from build123d import *

# Parameters (mm, degrees)
CUT_EXTRUDE_START   = -25
CUT_EXTRUDE_1_DEPTH = 25
SKETCH_3_W          = 3.2
SKETCH_3_H          = 16
CUT_EXTRUDE_2_DEPTH = 4
SKETCH_4_R          = 1.6
CUT_EXTRUDE_3_DEPTH = 10


with BuildPart() as part:
    # 草图1 → 旋转1 (revolve)
    with BuildSketch(Plane.XY, mode=Mode.PRIVATE) as revolve_1_sk:
        with BuildLine():
            Line((-16.340250108, 47.540513379), (-16.340250108, -2.459486621))
            Line((-16.340250108, -2.459486621), (-8.840250108, -2.459486621))
            Line((-8.840250108, -2.459486621), (-8.840250108, 32.540513379))
            Line((-8.840250108, 32.540513379), (-12.511021874, 44.696805356))
            ThreePointArc((-12.511021874, 44.696805356), (-13.955419706, 46.751834595), (-16.340250108, 47.540513379))
        make_face()
    revolve(revolve_1_sk.sketch.rotate(Axis((-16.340250108, 47.540513379, 0), (0, -1, 0)), 180), axis=Axis((-16.340250108, 47.540513379, 0), (0, -1, 0)))

    # 草图2 → 切除-拉伸1 (cut)
    with BuildSketch(Plane.XZ.offset(2.459486621).offset(CUT_EXTRUDE_START)):
        with BuildLine():
            Line((-21.930420052, 5), (-10.750080164, 5))
            ThreePointArc((-10.750080164, 5), (-16.340250108, 7.5), (-21.930420052, 5))
        make_face()
        with BuildLine():
            Line((-21.930420052, -5), (-10.750080164, -5))
            ThreePointArc((-10.750080164, -5), (-16.340250108, -7.5), (-21.930420052, -5))
        make_face()
    extrude(amount=CUT_EXTRUDE_1_DEPTH, mode=Mode.SUBTRACT)

    # 草图3 → 切除-拉伸2 (cut)
    with BuildSketch(Plane.XY.offset(5)):
        with Locations((-16.340250108, 14.540513379)):
            Rectangle(SKETCH_3_W, SKETCH_3_H)
    extrude(amount=-CUT_EXTRUDE_2_DEPTH, mode=Mode.SUBTRACT)

    # 草图4 → 切除-拉伸3 (cut)
    with BuildSketch(Plane.XY.offset(1)):
        with Locations((-16.340250108, 13.540513379)):
            Circle(SKETCH_4_R)
    extrude(amount=-CUT_EXTRUDE_3_DEPTH, mode=Mode.SUBTRACT)


solid = part.part
Model file for the job. Use its own axes, mm. A direction names the side the tool comes from. Coordinates: 2 decimals unless noted, no trailing zeros. Order: outer loops, then holes, each group sorted by start corner. A loop starts at its lowest first (then second) coordinate and runs counter-clockwise, first axis right, second up. Notation, with made-up numbers: M 49.25,-16 L 103.25,-16 A20 ccw 103.25,0 Z; hole C -18,31 d6. An arc over 180 degrees is marked long. Return JSON: item names as keys, results as strings.
1. Pull direction X, two halves, no side cores. Call faces 1 (the face through (-23.27, 19.17, 2.87)), 2 (the face through (-17.94, 14, 3)), 3 (the face through (-16, -2.459, 0)): +X half, -X half, draft (parallel to the pull), parting line (faces both ways), or undercut.
Ans:
{"face 1": "parting line", "face 2": "undercut", "face 3": "draft"}
2. Saw through at C-C (y = 40). Give the cut face in (x, z) (1 decimal).
Ans:
{"outline": "C -16.3,0 d10.5"}
3. Tool access for faces 4 (the face through (-11.114, 40.054, -0.23)), 5 (the face through (-16, 9, 1)), 6 (the face through (-16, 10, -5)), 7 (the face through (-19, 10, 5)): list every direction of +Z, -Z, +X, -X, +Y, -Y with a clear straight run to the whole face (end or side of a thin tool).
Ans:
{"face 4": "+Y", "face 5": "+Z", "face 6": "-Z, +X, -X, -Y", "face 7": "+Z, +X, -X, -Y"}
4. Saw through at B-B (y = 27). Give the cut face in (x, z).
Ans:
{"outline": "C -16.34,0 d15"}
5. Drill centre lines: probe 1 along Z at (x, y) = (-11.5, 8.5); probe 2 along X at (y, z) = (18, 4.25); probe 3 along X at (y, z) = (25, 3.5). Where is each one in solid material? Low to high.
Ans:
{"probe 1": "-5 to 5", "probe 2": "-22.52 to -17.94, -14.74 to -10.16", "probe 3": "-22.97 to -9.71"}
6. Flat gauge pins, fed straight in: pin 1 (1.6 mm diameter, centred on x = -17, y = 9, fed in from +Z); pin 2 (8 mm diameter, centred on x = -22, y = 3.5, fed in from -Z); pin 3 (4 mm diameter, centred on y = 8, z = -0.5, fed in from +X); pin 4 (3 mm diameter, centred on y = 39, z = -5, fed in from +X). Where does each tip first touch, or does it go through?
Ans:
{"pin 1": "z = 1", "pin 2": "z = -5", "pin 3": "x = -8.84", "pin 4": "x = -11.9"}
7. Saw through at A-A (z = 0). Give the cut face in (x, y), and give its area (3 significant figures).
Ans:
{"outline": "M -23.84,-2.46 L -8.84,-2.46 L -8.84,32.54 L -12.51,44.7 A4 ccw -20.17,44.7 L -23.84,32.54 Z; hole C -16.34,13.54 d3.2", "area": "671 mm^2"}
